```python
from build123d import *

# Parameters (mm, degrees)
FILLET1_R     = 1.524
CHAMFER1_SIZE = 0.762
CHAMFER2_SIZE = 0.762


with BuildPart() as part:
    # Sketch2 → Revolve1 (revolve)
    with BuildSketch(Plane.XY, mode=Mode.PRIVATE) as revolve1_sk:
        with BuildLine():
            Line((0, 0), (0, 41.275))
            ThreePointArc((0, 41.275), (-0.736350012, 40.709042493), (-0.378886857, 39.851873121))
            Line((-0.378886857, 39.851873121), (-4.064, 38.179030904))
            Line((-4.064, 38.179030904), (-6.946791529, 39.254381297))
            Line((-6.946791529, 39.254381297), (-4.572, 31.7246))
            Line((-4.572, 31.7246), (-6.096, 31.7246))
            Line((-6.096, 31.7246), (-6.096, 30.2006))
            Line((-6.096, 30.2006), (-6.858, 30.2006))
            ThreePointArc((-6.858, 30.2006), (-7.62, 29.4386), (-6.858, 28.6766))
            Line((-6.858, 28.6766), (-4.572, 28.6766))
            Line((-4.572, 28.6766), (-6.477, 4.699))
            Line((-6.477, 4.699), (-8.001, 4.699))
            Line((-8.001, 4.699), (-8.001, 3.175))
            Line((-8.001, 3.175), (-9.525, 3.175))
            Line((-9.525, 3.175), (-9.525, 0))
            Line((-9.525, 0), (0, 0))
        make_face()
    revolve(revolve1_sk.sketch.rotate(Axis((0, 0, 0), (0, 1, 0)), 270), axis=Axis((0, 0, 0), (0, 1, 0)))

    # Fillet1
    fillet1_edges = [part.edges().sort_by_distance(p)[0] for p in [
        (0, 4.699, 8.001),
    ]]
    fillet(fillet1_edges, radius=FILLET1_R - 0.0001)  # a hair under: the kernel refuses the full size

    # Chamfer1
    chamfer1_edges = [part.edges().sort_by_distance(p)[0] for p in [
        (0, 3.175, 9.525),
    ]]
    chamfer(chamfer1_edges, length=CHAMFER1_SIZE)

    # Chamfer2
    chamfer2_edges = [part.edges().sort_by_distance(p)[0] for p in [
        (0, 31.7246, 6.096),
    ]]
    chamfer(chamfer2_edges, length=CHAMFER2_SIZE)


solid = part.part
```
The model under review builds one solid part; all positions refer to its coordinate system, in mm. A direction names the side the tool comes from. Round coordinates to 2 decimals unless told otherwise and drop trailing zeros. Write each loop counter-clockwise with the first axis right and the second up, starting at its lowest first coordinate (ties: lowest second). Pieces come first, ordered by that corner, then holes. Notation, with made-up numbers: M -16.5,41.5 L 19.5,41.5 A21 cw 19.5,46.5 Z; hole C -37,77.25 d8. An arc over 180 degrees is marked long. Use CSV: the item, a comma, the result in double quotes. Start each with the question number.
(1) Tool access review of faces 4 (the face through (3, 3.175, 8)), 5 (the face through (4.5, 28.677, 1.6)), 6 (the face through (0, 0, 0)): name each direction out of +Z, -Z, +X, -X, +Y, -Y from which nothing blocks a thin tool from reaching the whole face with its end or side.
(2) The part is to be moulded in two halves that separate along Z. For faces 1 (the face through (4, 30.201, -5)), 2 (the face through (2.121, 16.52, -5.116)), 3 (the face through (-0.18, 39.75, -0.58)), say which applies: +Z half, -Z half, draft (parallel to the pull), parting line (faces both ways), or undercut.
(3) For line 1 along Y through (x, z) = (-5.5, 6.75) (3 decimals); line 2 along Z through (x, y) = (6.5, 4), list the stretches that pass through material, from the lowest coordinate up.
(4) Clearance check with flat-ended pins moving along their axes: P1, Ø2, axis at y = 6, z = 7.5, coming from the +X side; P2, Ø8, axis at x = -5.5, y = 16.5, coming from the -Z side; P3, Ø5, axis at x = -1, z = 5.5, coming from the +Y side; P4, Ø3, axis at x = -1, z = -2.5, coming from the +Y side. State where each tip first meets the part, or that it passes through.
(5) We need section B-B, the plane z = 4.75. State how many separate pieces and enclosed holes the cut face has, then the cut area to 3 significant figures.
(6) We need section C-C, the plane y = 7. State the section outline as (x, z) points, then the cut area to 3 significant figures.
(7) We need section D-D, the plane y = 21. State the section outline as (x, z) points, then the cut area to 3 significant figures.
Findings:
1,face 4,"+Y"
1,face 5,"none"
1,face 6,"+Z, -Z, +X, -X, -Y"
2,face 1,"draft"
2,face 2,"parting line"
2,face 3,"undercut"
3,line 1,"0 to 3.175"
3,line 2,"-4.24 to 4.24"
4,P1,"through"
4,P2,"z = -5.38"
4,P3,"y = 39.25"
4,P4,"y = 39.48"
5,separate pieces,"3"
5,enclosed holes,"0"
5,area,"262 mm^2"
6,outline,"C 0,0 d12.59"
6,area,"124 mm^2"
7,outline,"C 0,0 d10.36"
7,area,"84.4 mm^2"
